Autodesk Fusion 360 part; units mm, degrees
sketch "Sketch1" plane through (0, 0, 0) normal (0, 0, 1) x (1, 0, 0) in component "Case"
  line L0 (0, 0) -> (42.9, 0)
  line L1 (42.9, 0) -> (42.9, 64.3)
  line L2 (42.9, 64.3) -> (0, 64.3)
  line L3 (0, 64.3) -> (0, 0)
  line L4 (53.4, 73.8) -> (-9.5, 73.8)
  line L5 (-9.5, 73.8) -> (-9.5, -8.5)
  line L6 (-9.5, -8.5) -> (53.4, -8.5)
  line L7 (53.4, -8.5) -> (53.4, 73.8)
  circle A0 centre (-4.5, 68.8) radius 1.7
  circle A1 centre (48.4, 68.8) radius 1.7
  circle A2 centre (48.4, -3.5) radius 1.7
  circle A3 centre (-4.5, -3.5) radius 1.7
  circle A4 centre (48.4, 68.8) radius 3
  circle A5 centre (48.4, -3.5) radius 3
  circle A6 centre (-4.5, 68.8) radius 3
  circle A7 centre (-4.5, -3.5) radius 3
  dimension "d1" = 42.9
  dimension "d2" = 64.3
  dimension "d3" = 62.9
  dimension "d4" = 82.3
  dimension "d5" = 9.5
  dimension "d6" = 9.5
  dimension "d7" = 3.4
  dimension "d8" = 3.4
  dimension "d9" = 3.4
  dimension "d10" = 3.4
  dimension "d11" = 5
  dimension "d12" = 5
  dimension "d13" = 5
  dimension "d14" = 5
  dimension "d15" = 5
  dimension "d16" = 5
  dimension "d17" = 5
  dimension "d18" = 5
  dimension "d19" = 1.3
  dimension "d20" = 1.3
  dimension "d21" = 1.3
  dimension "d22" = 1.3
extrude "Extrude1" add sketch "Sketch1" along normal blind 9.9 from surface at 3.1 contours A4 | A5 | A6 | A7 makes body 1 at (51.3963, -3.6495, 9.7) makes body 2 at (50.9599, 70.3643, 9.7) makes body 3 at (-1.5037, -3.6495, 9.7) makes body 4 at (-7.0599, 67.2357, 9.7) in component "Case"
extrude "Extrude2" add sketch "Sketch1" along normal blind 13 contours L4 L5 L6 L7 bodies 1 2 3 4 in component "Case"
extrude "Extrude3" add sketch "Sketch1" along normal blind 3 contours L0 L1 L2 L3 bodies 1 in component "Case"
sketch "Sketch2" plane through (0, 0, 13) normal (0, 0, 1) x (-1, 0, 0) in component "Case"
  circle A0 centre (-48.4, 3.5) radius 1.7
  circle A1 centre (4.5, -68.8) radius 1.7
  line L0 (0, 0) -> (0, -64.3)
  line L1 (0, -64.3) -> (-42.9, -64.3)
  line L2 (-42.9, -64.3) -> (-42.9, 0)
  line L3 (-42.9, 0) -> (0, 0)
  line L4 (-53.4, 8.5) -> (-53.4, -73.8)
  line L5 (-53.4, -73.8) -> (9.5, -73.8)
  line L6 (9.5, -73.8) -> (9.5, 8.5)
  line L7 (9.5, 8.5) -> (-53.4, 8.5)
  circle A2 centre (-48.4, -68.8) radius 1.7
  circle A3 centre (4.5, 3.5) radius 1.7
  line L8 (0, -64.3) -> (0, 0)
  line L9 (0, 0) -> (-42.9, 0)
  line L10 (-42.9, 0) -> (-42.9, -64.3)
  line L11 (-42.9, -64.3) -> (0, -64.3)
  line L12 (-10.71, -73.8) -> (-29.21, -73.8)
  line L13 (-29.21, -73.8) -> (-29.21, -64.3)
  line L14 (-29.21, -64.3) -> (-10.71, -64.3)
  line L15 (-10.71, -64.3) -> (-10.71, -73.8)
  dimension "d31" = 10.71
  dimension "d32" = 13.69
extrude "Extrude4" cut sketch "Sketch2" against normal blind 10 contours L1 L5 L11 L12 L13 L14 L15 bodies 1 in component "Case"
component "Case" placed x (1, 0, 0) y (0, 1, 0) z (0, 0, 1) at (0, 0, 0)
equation "d31 = 14.46 mm - 3.75 mm"
equation "d32 = 14.46 mm - 0.77 mm"
Input: part model. Units: mm. Frame: model coordinates. A direction names the side the tool comes from. Give positions to 0.01 mm unless a question says otherwise; leave off trailing zeros. Order: outer loops, then holes, each group sorted by start corner. A loop starts at its lowest first (then second) coordinate and runs counter-clockwise, first axis right, second up. Notation, with made-up numbers: (78.5, 87.5) - (100.5, 87.5) arc R17 cw to (100.5, 102.5) - close; hole circle Ø9 at (32, 71). An arc over 180 degrees is marked (long way). One line per item, written item: value.
1. Cut plane A-A, the plane x = -4.5. Output: boundary loops of the cut face in (y, z).
Determined:
outline: (-8.5, 0) - (-6.5, 0) - (-6.5, 3.1) - (-5.2, 3.1) - (-5.2, 13) - (-8.5, 13) - close; (-1.8, 3.1) - (-0.5, 3.1) - (-0.5, 0) - (65.8, 0) - (65.8, 3.1) - (67.1, 3.1) - (67.1, 13) - (-1.8, 13) - close; (70.5, 3.1) - (71.8, 3.1) - (71.8, 0) - (73.8, 0) - (73.8, 13) - (70.5, 13) - close
2. Reachability of faces 4 (the face through (-3, -5, 3.1)), 5 (the face through (0, 33, 8)), 6 (the face through (10.71, 69, 8)) from +Z, -Z, +X, -X, +Y, -Y: full face, straight path, thin tool, end or side. Return the list, or none.
Determined:
face 4: -Z
face 5: +Z
face 6: +Z, +Y
3. Cut plane D-D, the plane x = 41. Output: boundary loops of the cut face in (y, z).
Determined:
outline: (-8.5, 0) - (73.8, 0) - (73.8, 13) - (64.3, 13) - (64.3, 3) - (0, 3) - (0, 13) - (-8.5, 13) - close
4. Pin query (flat end, axial travel): pin 1 Ø1.8 at (x, y) = (49.5, 68.5) entering from -Z; pin 2 Ø2 at (x, z) = (15.5, 9.5) entering from +Y; pin 3 Ø8 at (x, y) = (37.5, 28) entering from +Z. Return the tip coordinate at first contact, or that it passes through.
Determined:
pin 1: z = 3.1
pin 2: y = 0
pin 3: z = 3
5. Draft query along X for faces 1 (the face through (5, 64.3, 8)), 2 (the face through (-5, 67, 3.1)), 3 (the face through (22, 33, 0)). Return one class per face: released by +X, released by -X, zero draft, split by the parting line, or undercut.
Determined:
face 1: undercut
face 2: undercut
face 3: zero draft
6. Cut plane C-C, the plane z = 5.25. Output: boundary loops of the cut face in (x, y).
Determined:
outline: (-9.5, -8.5) - (53.4, -8.5) - (53.4, 73.8) - (29.21, 73.8) - (29.21, 64.3) - (42.9, 64.3) - (42.9, 0) - (0, 0) - (0, 64.3) - (10.71, 64.3) - (10.71, 73.8) - (-9.5, 73.8) - close; hole circle Ø3.4 at (-4.5, -3.5); hole circle Ø3.4 at (-4.5, 68.8); hole circle Ø3.4 at (48.4, -3.5); hole circle Ø3.4 at (48.4, 68.8)
7. Line query: probe 1 along Y at (x, z) = (-4.5, 5.5); probe 2 along Y at (x, z) = (48.4, 1); probe 3 along X at (y, z) = (68.8, 7.5). Output: solid intervals per line, ascending.
Determined:
probe 1: -8.5 to -5.2, -1.8 to 67.1, 70.5 to 73.8
probe 2: -8.5 to -6.5, -0.5 to 65.8, 71.8 to 73.8
probe 3: -9.5 to -6.2, -2.8 to 10.71, 29.21 to 46.7, 50.1 to 53.4
8. Cut plane B-B, the plane y = 68.8. Output: boundary loops of the cut face in (x, z), and give its area (3 significant figures).
Determined:
outline: (-9.5, 0) - (-7.5, 0) - (-7.5, 3.1) - (-6.2, 3.1) - (-6.2, 13) - (-9.5, 13) - close; (-2.8, 3.1) - (-1.5, 3.1) - (-1.5, 0) - (45.4, 0) - (45.4, 3.1) - (46.7, 3.1) - (46.7, 13) - (29.21, 13) - (29.21, 3) - (10.71, 3) - (10.71, 13) - (-2.8, 13) - close; (50.1, 3.1) - (51.4, 3.1) - (51.4, 0) - (53.4, 0) - (53.4, 13) - (50.1, 13) - close
area: 528 mm2
